The model under review builds one solid part; all positions refer to its coordinate system, in mm. Face numbers are marked on the shaded views. Round coordinates to 2 decimals unless told otherwise and drop trailing zeros. Loops run counter-clockwise (first coordinate to the right, second up) from the corner with the lowest first, then second, coordinate; pieces in that order, holes last. Notation, with made-up numbers: (16, 59.5) -> (31, 59.5) arc R24 ccw to (31, 74.5) -> close; hole circle Ø7 at (52, 46.5). An arc over 180 degrees is marked (long way). Return JSON: item names as keys, results as strings. Group by question number.
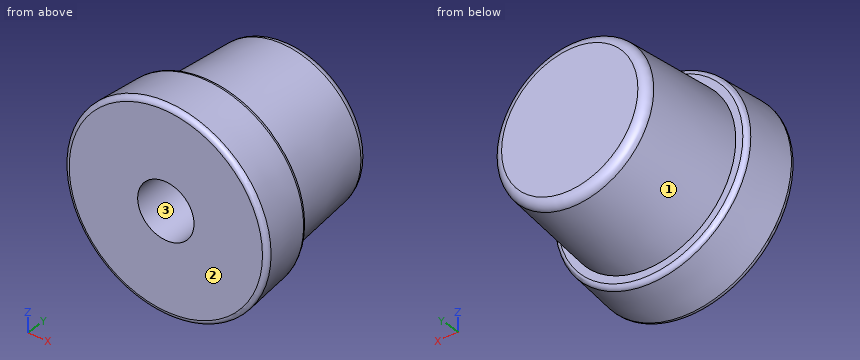
```python
from build123d import *

# Parameters (mm, degrees)
SKETCH1_R           = 11
BOSS_EXTRUDE1_DEPTH = 6
BOSS_EXTRUDE1_TAPER = 5
SKETCH2_R           = 9.25
BOSS_EXTRUDE2_DEPTH = 11
BOSS_EXTRUDE2_TAPER = 5
SKETCH3_R           = 3.05
CUT_EXTRUDE1_DEPTH  = 8
FILLET1_R           = 1
FILLET2_R           = 0.5
FILLET3_R           = 0.5


with BuildPart() as part:
    # Sketch1 → Boss-Extrude1 (new body)
    with BuildSketch(Plane(origin=(0, 0, 0), x_dir=(1, 0, 0), z_dir=(0, 1, 0))):
        Circle(SKETCH1_R)
    extrude(amount=BOSS_EXTRUDE1_DEPTH, taper=BOSS_EXTRUDE1_TAPER)

    # Sketch2 → Boss-Extrude2 (add)
    with BuildSketch(Plane(origin=(0, 6, 0), x_dir=(1, 0, 0), z_dir=(0, 1, 0))):
        Circle(SKETCH2_R)
    extrude(amount=BOSS_EXTRUDE2_DEPTH, taper=BOSS_EXTRUDE2_TAPER)

    # Sketch3 → Cut-Extrude1 (cut)
    with BuildSketch(Plane.XZ):
        with Locations(Location((0, 0, 0), (0, 0, 270))):
            Circle(SKETCH3_R)
    extrude(amount=-CUT_EXTRUDE1_DEPTH, mode=Mode.SUBTRACT)

    # Fillet1
    fillet1_edges = [part.edges().sort_by_distance(p)[0] for p in [
        (-8.287624701, 17, 0),
    ]]
    fillet(fillet1_edges, radius=FILLET1_R)

    # Fillet2
    fillet2_edges = [part.edges().sort_by_distance(p)[0] for p in [
        (-10.475068019, 6, 0),
    ]]
    fillet(fillet2_edges, radius=FILLET2_R)

    # Fillet3
    fillet3_edges = [part.edges().sort_by_distance(p)[0] for p in [
        (-11, 0, 0),
    ]]
    fillet(fillet3_edges, radius=FILLET3_R)


solid = part.part
```
1. We need section C-C, the plane y = 14.5. Write out the cut boundary in (x, z).
2. We need section A-A, the plane x = 0. Write out the cut boundary in (y, z) (3 decimals).
3. For P1, Ø2, axis at x = -7.5, y = 6, coming from the -Z side; P2, Ø4, axis at y = 3.5, z = 3.5, coming from the +X side; P3, Ø2, axis at y = 13, z = 0.5, coming from the +X side, all flat-tipped, find the tip position at first contact; note any pin that passes through.
4. Wall thickness on line 1 (Y direction, x = 8.75, z = -4.75); line 2 (X direction, y = 6.25, z = 0); line 3 (X direction, y = 2, z = 0.75): over which ranges is each line inside the solid? List them lowest first.
5. We need section B-B, the plane y = 11. Write out the cut boundary in (x, z), then the cut area to 3 significant figures.
6. Draft analysis for pull direction Z (two halves, no side actions). For the marked faces 1, 2 and 3, state which applies: pulls with the +Z half, pulls with the -Z half, needs draft (parallel to the pull), parting line crosses it, or undercut.
Check sheet entries:
{
 "1": {"outline": "circle Ø17.01 at (0, 0)"},
 "2": {"outline": "(0, -10.454) arc R0.5 ccw to (0.544, -10.952) -> (5.544, -10.515) arc R0.5 ccw to (6, -10.017) -> (6, -9.25) -> (16.087, -8.367) arc R1 ccw to (17, -7.371) -> (17, 7.371) arc R1 ccw to (16.087, 8.367) -> (6, 9.25) -> (6, 10.017) arc R0.5 ccw to (5.544, 10.515) -> (0.544, 10.952) arc R0.5 ccw to (0, 10.454) -> (0, 3.05) -> (8, 3.05) -> (8, -3.05) -> (0, -3.05) -> close"},
 "3": {"P1": "stops at z = -8.19", "P2": "stops at x = 10.64", "P3": "stops at x = 8.72"},
 "4": {"line 1": "y = 0 to 6", "line 2": "x = -9.23 to -3.05, 3.05 to 9.23", "line 3": "x = -10.8 to -2.96, 2.96 to 10.8"},
 "5": {"outline": "circle Ø17.63 at (0, 0)", "area": "244 mm²"},
 "6": {"face 1": "parting line crosses it", "face 2": "needs draft", "face 3": "undercut"}
}
